Model file for the job. Use its own axes, mm. A direction names the side the tool comes from. Give positions to 0.01 mm unless a question says otherwise; leave off trailing zeros. Loops run counter-clockwise (first coordinate to the right, second up) from the corner with the lowest first, then second, coordinate; pieces in that order, holes last. Notation, with made-up numbers: M 51.25,-38 L 74.25,-38 A20 ccw 74.25,-15 Z; hole C 40.25,-34.5 d5. An arc over 180 degrees is marked long. Answer in a Markdown table with one row per item.
Autodesk Inventor part; units mm, degrees
ref_plane "YZ Plane" through (0, 0, 0) normal (1, 0, 0) x (0, 1, 0)
ref_plane "XZ Plane" through (0, 0, 0) normal (0, 1, 0) x (-1, 0, 0)
ref_plane "XY Plane" through (0, 0, 0) normal (0, 0, 1) x (1, 0, 0)
sketch "Sketch1" plane through (0, 0, 0) normal (0, 1, 0) x (-1, 0, 0)
  line L0 (17.5, 17.5) -> (-17.5, 17.5)
  line L1 (-17.5, 17.5) -> (-17.5, -17.5)
  line L2 (-17.5, -17.5) -> (17.5, -17.5)
  line L3 (17.5, -17.5) -> (17.5, 17.5)
  line L4 (17.5, 17.5) -> (-17.5, -17.5) construction
  line L5 (-17.5, 17.5) -> (17.5, -17.5) construction
  point P0 (0, 0)
  dimension "d0" = 35
  dimension "d1" = 35
extrude "Extrusion1" add sketch "Sketch1" along normal mid plane 25
sketch "Sketch2" plane through (0, 12.5, 0) normal (0, 1, 0) x (1, 0, 0)
  circle A0 centre (0, 0) radius 4.15
  dimension "d4" = 8.3
extrude "Extrusion2" cut sketch "Sketch2" against normal blind 25
sketch "Sketch3" plane through (0, 12.5, 0) normal (0, 1, 0) x (1, 0, 0)
  circle A0 centre (0, 0) radius 11.25
  dimension "d7" = 22.5
extrude "Extrusion3" cut sketch "Sketch3" against normal blind 11
sketch "Sketch4" plane through (0, 12.5, 0) normal (0, 1, 0) x (1, 0, 0)
  circle A0 centre (0, 0) radius 4.15
  circle A1 centre (0, 0) radius 16
  line L0 (17.5, 17.5) -> (-17.5, 17.5)
  line L1 (-17.5, -17.5) -> (17.5, -17.5)
  line L2 (17.5, 17.5) -> (-17.5, -17.5)
  line L3 (-17.5, 17.5) -> (17.5, -17.5)
  circle A2 centre (11.3137, 11.3137) radius 1.65
  circle A3 centre (-11.3137, 11.3137) radius 1.65
  circle A4 centre (-11.3137, -11.3137) radius 1.65
  circle A5 centre (11.3137, -11.3137) radius 1.65
  dimension "d10" = 32
  dimension "d11" = 3.3
  dimension "d14" = 360
extrude "Extrusion4" cut sketch "Sketch4" against normal blind 25 contours A2 A1 L2 | L2 A1 A2 | A5 A1 L3 | L3 A1 A5 | A3 A1 L3 | L3 A1 A3 | L2 A2 A1 | A1 A2 L2 | A4 A1 L2 | L2 A1 A4 | L3 A5 A1 | A1 A5 L3 | L3 A3 A1 | A1 A3 L3 | L2 A4 A1 | A1 A4 L2
fillet "Fillet1" radius 9 2 edges at (-17.5, 0, -17.5) (-17.5, 0, 17.5)
mirror "Mirror1" about plane through (0, 0, 0) normal (0, 1, 0) of "Extrusion3"
properties part number "PART_!"
Q1. Mould opens along Z. For faces 4 (the face through (-17.5, 0, 0)), 5 (the face through (12.2, 0.18, 9.92)), 6 (the face through (0, 1.5, 5)), 7 (the face through (5, 0, -17.5)) say: released by +Z, released by -Z, zero draft, split by the parting line, or undercut.
Reported:
| item | result |
|---|---|
| face 4 | zero draft |
| face 5 | undercut |
| face 6 | undercut |
| face 7 | released by -Z |
Q2. Saw through at B-B (x = 0). Give the cut face in (y, z).
Reported:
| item | result |
|---|---|
| outline | M -12.5,-17.5 L 12.5,-17.5 L 12.5,-11.25 L 1.5,-11.25 L 1.5,-4.15 L -1.5,-4.15 L -1.5,-11.25 L -12.5,-11.25 Z; M -12.5,11.25 L -1.5,11.25 L -1.5,4.15 L 1.5,4.15 L 1.5,11.25 L 12.5,11.25 L 12.5,17.5 L -12.5,17.5 Z |
Q3. Saw through at D-D (x = -9). Give the cut face in (y, z), and give its area (3 significant figures).
Reported:
| item | result |
|---|---|
| outline | M -12.5,-17.49 L 12.5,-17.49 L 12.5,-6.75 L 1.5,-6.75 L 1.5,6.75 L 12.5,6.75 L 12.5,17.49 L -12.5,17.49 L -12.5,6.75 L -1.5,6.75 L -1.5,-6.75 L -12.5,-6.75 Z |
| area | 577 mm² |
Q4. Saw through at C-C (y = 0). Give the cut face in (x, z), and give its area (3 significant figures).
Reported:
| item | result |
|---|---|
| outline | M -17.5,-8.5 A9 ccw -8.5,-17.5 L 17.5,-17.5 L 17.5,17.5 L -8.5,17.5 A9 ccw -17.5,8.5 Z; hole C -11.31,-11.31 d3.3; hole C -11.31,11.31 d3.3; hole C 0,0 d8.3; hole C 11.31,-11.31 d3.3; hole C 11.31,11.31 d3.3 |
| area | 1,100 mm² |
Q5. Probe probe 1 along Z at (x, y) = (0, 5.5); probe 2 along X at (y, z) = (3.25, -12); probe 3 along X at (y, z) = (10.5, -10). List the from-to ranges inside material, lowest first.
Reported:
| item | result |
|---|---|
| probe 1 | -17.5 to -11.25, 11.25 to 17.5 |
| probe 2 | -16.79 to -12.81, -9.81 to 9.81, 12.81 to 17.5 |
| probe 3 | -17.37 to -12.31, -10.32 to -5.15, 5.15 to 10.32, 12.31 to 17.5 |
Q6. 3-axis set-ups, long thin cutter, end or side, ignore diameter. For faces 1 (the face through (4, 0, 17.5)), 2 (the face through (0, -1.5, 5)), 3 (the face through (5.19, 7.08, 9.98)): which of +Z, -Z, +X, -X, +Y, -Y reach the whole face in a straight line?
Reported:
| item | result |
|---|---|
| face 1 | +Z, +X, -X, +Y, -Y |
| face 2 | -Y |
| face 3 | +Y |
Q7. Saw through at A-A (z = 0). Give the cut face in (x, y).
Reported:
| item | result |
|---|---|
| outline | M -17.5,-12.5 L -11.25,-12.5 L -11.25,-1.5 L -4.15,-1.5 L -4.15,1.5 L -11.25,1.5 L -11.25,12.5 L -17.5,12.5 Z; M 4.15,-1.5 L 11.25,-1.5 L 11.25,-12.5 L 17.5,-12.5 L 17.5,12.5 L 11.25,12.5 L 11.25,1.5 L 4.15,1.5 Z |
Q8. Drop flat-ended pins along their axis: pin 1 (3 mm diameter, centred on x = -11.31, z = -11.31, fed in from -Y); pin 2 (1.5 mm diameter, centred on y = -2.5, z = 10.5, fed in from -X); pin 3 (6 mm diameter, centred on x = -2.5, z = 5.5, fed in from -Y); pin 4 (20 mm diameter, centred on x = 0, z = 0, fed in from +Y). Give the stop position or say it passes through.
Reported:
| item | result |
|---|---|
| pin 1 | through |
| pin 2 | x = -17.41 |
| pin 3 | y = -1.5 |
| pin 4 | y = 1.5 |
